The listing builds one solid part. Answer for the finished solid, in the listing's coordinates (mm). A direction names the side the tool comes from. Coordinates: 2 decimals unless noted, no trailing zeros. Loops run counter-clockwise (first coordinate to the right, second up) from the corner with the lowest first, then second, coordinate; pieces in that order, holes last. Notation, with made-up numbers: M 35.25,73.5 L 56.25,73.5 A20 cw 56.25,90.5 Z; hole C 87,13.25 d2. An arc over 180 degrees is marked long. Return JSON: item names as keys, results as strings. Group by question number.
1. Section D-D (x = -28.5) is taken. Write down the section's boundary in (y, z) (1 decimal), then the cut area to 3 significant figures.
2. Given P1, Ø6, axis at x = -34, y = -40.5, coming from the -Z side; P2, Ø12.5, axis at x = 5, y = -30, coming from the +Z side; P3, Ø12, axis at x = 40, y = -41.5, coming from the +Z side, each flat-ended and moving along its own axis, determine where each tip first touches the part or whether it passes through.
3. The mould has two halves that part along Z. Classify faces 4 (the face through (12.7, -25, 0)), 5 (the face through (-13.77, -25.04, -61.99)), 6 (the face through (-31.75, -8, 0)), 7 (the face through (13, 0, 1)): pulls with the +Z half, pulls with the -Z half, needs draft (parallel to the pull), parting line crosses it, or undercut.
4. Straight lines are drawn through the part: L1, parallel to Y at x = -23, z = -1; L2, parallel to Z at x = -16, y = -8.5; L3, parallel to Z at x = 8.5, y = -17. For each, find the intervals that lie inside material, in ascending order. Write a range as from..to.
5. Which of the six approach directions +Z, -Z, +X, -X, +Y, -Y give full straight-line access (tool end or side, diameter ignored) to faces 1 (the face through (-22.092, -9.285, 0.07)), 2 (the face through (13, -50.8, 1)), 3 (the face through (0, -25, 12.7))?
6. Section B-B (z = 0) is taken. Write down the section's boundary in (x, y).
7. Section C-C (y = -32) is taken. Write down the section's boundary in (x, z).
8. Section A-A (x = 0) is taken. Write down the section's boundary in (y, z), then the cut area to 3 significant figures.
```python
from build123d import *

# Parameters (mm, degrees)
F0_R     = 63.5
F1_DEPTH = 50.8
F2_W     = 25.4
F2_H     = 25.4
F3_DEPTH = 50.8
F4_R     = 1.5875
F5_DEPTH = 31.75


with BuildPart() as f1:
    # F0 (on Front) → F1 (new body)
    with BuildSketch(Plane.XZ):
        Circle(F0_R)
    extrude(amount=F1_DEPTH)

    # F2 (on face) → F3 (cut)
    with BuildSketch(Plane(origin=(0, 0, 0), x_dir=(-1, 0, 0), z_dir=(0, 1, 0))):
        Rectangle(F2_W, F2_H)
    extrude(amount=-F3_DEPTH, mode=Mode.SUBTRACT)

    # F4 (on Right) → F5 (cut)
    with BuildSketch(Plane.YZ):
        with Locations((-7.698557, 0)):
            Circle(F4_R)
    extrude(amount=-F5_DEPTH, mode=Mode.SUBTRACT)


solid = f1.part
```
Worked out:
{
 "1": {"outline": "M -50.8,-56.7 L 0,-56.7 L 0,56.7 L -50.8,56.7 Z; hole C -7.7,0 d3.2", "area": "5,760 mm^2"},
 "2": {"P1": "z = -55.42", "P2": "z = 63.5", "P3": "z = 53.63"},
 "3": {"face 4": "undercut", "face 5": "parting line crosses it", "face 6": "undercut", "face 7": "needs draft"},
 "4": {"L1": "-50.8..-8.93, -6.47..0", "L2": "-61.45..-1.37, 1.37..61.45", "L3": "-62.93..-12.7, 12.7..62.93"},
 "5": {"face 1": "none", "face 2": "+Z, -Z, +X, -X, -Y", "face 3": "+Y, -Y"},
 "6": {"outline": "M -63.5,-50.8 L -12.7,-50.8 L -12.7,-9.29 L -31.75,-9.29 L -31.75,-6.11 L -12.7,-6.11 L -12.7,0 L -63.5,0 Z; M 12.7,-50.8 L 63.5,-50.8 L 63.5,0 L 12.7,0 Z"},
 "7": {"outline": "C 0,0 d127; hole M -12.7,-12.7 L 12.7,-12.7 L 12.7,12.7 L -12.7,12.7 Z"},
 "8": {"outline": "M -50.8,-63.5 L 0,-63.5 L 0,-12.7 L -50.8,-12.7 Z; M -50.8,12.7 L 0,12.7 L 0,63.5 L -50.8,63.5 Z", "area": "5,160 mm^2"}
}
